Can you work these out from the model? Positions are in its coordinate system, mm. A direction names the side the tool comes from. Coordinates: 2 decimals unless noted, no trailing zeros. Order: outer loops, then holes, each group sorted by start corner. A loop starts at its lowest first (then second) coordinate and runs counter-clockwise, first axis right, second up. Notation, with made-up numbers: (9.5, 69) -> (32.5, 69) arc R25 cw to (32.5, 86) -> close; hole circle Ø3 at (20, 88.5). An arc over 180 degrees is marked (long way). Return JSON: item names as keys, results as strings. Group by question number.
1) Thinking about a two-plate mould opening in X: for faces 1 (the flat face through (2.858, 10, 0)), 2 (the flat face through (15.875, -11, 0)), 3 (the cylindrical face through (4.262, -10.074, -1.323)), which applies, +X half, -X half, draft (parallel to the pull), parting line (faces both ways), or undercut?
2) For faces 4 (the flat face through (0, -11, 0)), 5 (the flat face through (4.762, 7, 7)), 6 (the cylindrical face through (2.91, -9.57, -1.26)), 7 (the flat face through (13.018, 10, 0)), which set-ups out of +Z, -Z, +X, -X, +Y, -Y let a thin tool reach every point of the face, with its end or its side?
3) If I drill on probe 1 along Y at (x, z) = (4.4, 0); probe 2 along Y at (x, z) = (7.5, 0); probe 3 along Z at (x, y) = (8.5, 0.25), over which ranges is the centre line in solid material (lowest first)? Write a range as from..to.
4) If we section it at B-B, the plane y = 0: Please give me the cut outline in (x, z).
5) If we section it at C-C, the plane x = 4.25: Please give me the cut outline in (y, z).
6) For pin 1 (6 mm diameter, centred on x = 12.5, z = -3, fed in from -Y); pin 2 (1 mm diameter, centred on y = -1, z = -8.5, fed in from -X); pin 3 (9 mm diameter, centred on y = 4, z = -3, fed in from +X); pin 4 (1.5 mm diameter, centred on y = 4.5, z = 4, fed in from +X), each with a flat end and sliding along its axis, tell me the tip position at first contact or that it passes through.
from build123d import *

# Parameters (mm, degrees)
CUT_EXTRUDE1_DEPTH      = 24.970724332
CUT_EXTRUDE1_DEPTH_BACK = 24.970724332


with BuildPart() as part:
    # Sketch2 → Revolve1 (revolve)
    with BuildSketch(Plane(origin=(0, 0, 0), x_dir=(1, 0, 0), z_dir=(0, 1, 0)), mode=Mode.PRIVATE) as revolve1_sk:
        Polygon((4.7625, 9.398), (11.1125, 9.398), (11.1125, 8.636), (15.875, 8.636), (15.875, 12.7), (0, 12.7), (0, 9.652), (3.7465, 9.652), (3.7465, 10.16), (4.7625, 10.16), align=None)
    revolve(revolve1_sk.sketch.rotate(Axis((0, 0, 0), (1, 0, 0)), 180), axis=Axis((0, 0, 0), (1, 0, 0)))

    # Sketch6 → Cut-Extrude1 (cut, two sides: drawn at the far end of the back side and taken through both)
    with BuildSketch(Plane.XY.offset(-CUT_EXTRUDE1_DEPTH_BACK)):
        with BuildLine():
            Line((0, 12.7), (0, -10.16))
            ThreePointArc((0, -10.16), (2.097664354, -7.868773916), (2.8575, -4.856704444))
            Line((2.8575, -4.856704444), (2.8575, 12.7))
            Line((2.8575, 12.7), (0, 12.7))
        make_face()
        with BuildLine():
            ThreePointArc((15.875, -10.16), (13.777335646, -7.868773916), (13.0175, -4.856704444))
            Line((13.0175, -4.856704444), (13.0175, 12.7))
            Line((13.0175, 12.7), (15.875, 12.7))
            Line((15.875, 12.7), (15.875, -10.16))
        make_face()
    extrude(amount=CUT_EXTRUDE1_DEPTH + CUT_EXTRUDE1_DEPTH_BACK, mode=Mode.SUBTRACT)


solid = part.part
Result sheet:
{
 "1": {"face 1": "-X half", "face 2": "+X half", "face 3": "undercut"},
 "2": {"face 4": "+Z, -Z, -X, +Y, -Y", "face 5": "none", "face 6": "-X", "face 7": "+Z, -Z, +X, +Y"},
 "3": {"probe 1": "y = -12.7..-10.16, 10.16..12.7", "probe 2": "y = -12.7..-9.4, 9.4..12.7", "probe 3": "z = -12.7..-9.39, 9.39..12.7"},
 "4": {"outline": "(2.86, -12.7) -> (13.02, -12.7) -> (13.02, -8.64) -> (11.11, -8.64) -> (11.11, -9.4) -> (4.76, -9.4) -> (4.76, -10.16) -> (3.75, -10.16) -> (3.75, -9.65) -> (2.86, -9.65) -> close; (2.86, 9.65) -> (3.75, 9.65) -> (3.75, 10.16) -> (4.76, 10.16) -> (4.76, 9.4) -> (11.11, 9.4) -> (11.11, 8.64) -> (13.02, 8.64) -> (13.02, 12.7) -> (2.86, 12.7) -> close"},
 "5": {"outline": "circle Ø25.4 at (0, 0); hole circle Ø20.32 at (0, 0)"},
 "6": {"pin 1": "stops at y = -12.7", "pin 2": "stops at x = 11.11", "pin 3": "stops at x = 13.02", "pin 4": "passes through"}
}
